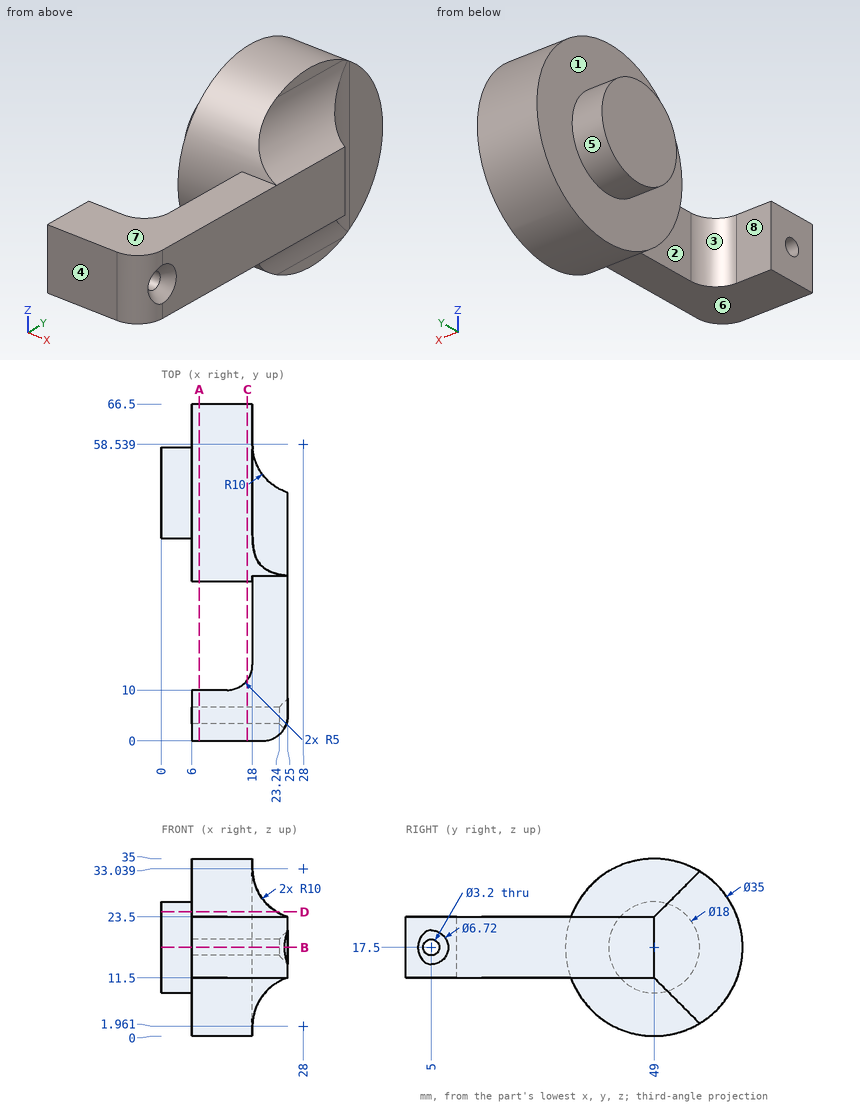
Source: three-view drawing plus pictorial views. Frame: mm from the lowest corner of the part. A direction names the side the tool comes from. Coordinates: 2 decimals unless noted, no trailing zeros. Order: outer loops, then holes, each group sorted by start corner. A loop starts at its lowest first (then second) coordinate and runs counter-clockwise, first axis right, second up. Notation, with made-up numbers: M -9,16 L 49,16 A27 ccw 49,41 Z; hole C 23,51 d9. An arc over 180 degrees is marked long. Answer in a Markdown table with one row per item.
(1) Section query D-D, the plane z = 24.5. Output: boundary loops of the cut face in (x, y).
Numbers:
| item | result |
|---|---|
| outline | M 0,43.34 L 6,43.34 L 6,32.96 L 22.8,32.96 L 22.8,50 A10 cw 18,58.54 L 18,65.04 L 6,65.04 L 6,54.66 L 0,54.66 Z |
(2) Draft query along Y for the marked faces 1, 2, 3 and 4. Return one class per face: pulls with the +Y half, pulls with the -Y half, needs draft (parallel to the pull), parting line crosses it, or undercut.
Numbers:
| item | result |
|---|---|
| face 1 | needs draft |
| face 2 | undercut |
| face 3 | undercut |
| face 4 | pulls with the -Y half |
(3) Section query C-C, the plane x = 17. Output: boundary loops of the cut face in (y, z), plus the area to 3 significant figures.
Numbers:
| item | result |
|---|---|
| outline | M 0,11.5 L 12,11.5 L 12,23.5 L 0,23.5 Z; C 49,17.5 d35; hole C 5,17.5 d3.2 |
| area | 1,100 mm^2 |
(4) Material intervals for line 1 (X direction, y = 59.5, z = 31); line 2 (Y direction, x = 3.25, z = 21.5); line 3 (X direction, y = 24.5, z = 17.5), sorted ascending. Write a range as [from, to].
Numbers:
| item | result |
|---|---|
| line 1 | x = [6, 18] |
| line 2 | y = [40.94, 57.06] |
| line 3 | x = [18, 25] |
(5) Section query B-B, the plane z = 17.5. Output: boundary loops of the cut face in (x, y).
Numbers:
| item | result |
|---|---|
| outline | M 0,40 L 6,40 L 6,31.5 L 18,31.5 L 18,15 A5 cw 13,10 L 6,10 L 6,6.6 L 23.24,6.6 L 25,8.36 L 25,49 A10 cw 18,58.54 L 18,66.5 L 6,66.5 L 6,58 L 0,58 Z; M 6,0 L 20,0 A5 ccw 24.26,2.38 L 23.24,3.4 L 6,3.4 Z |
(6) Access query for the marked faces 5, 6, 7 and 8. Directions: +Z, -Z, +X, -X, +Y, -Y. A direction counts if a zero-diameter tool reaches every point of the face in a straight line with its end or side. Return the directions, or none.
Numbers:
| item | result |
|---|---|
| face 5 | -X |
| face 6 | -Z, +X, -X, -Y |
| face 7 | +Z, +X, -X, -Y |
| face 8 | +Z, -Z, -X |
(7) Contact query for flat-ended pins moving along their axis: pin 1 Ø4 at (y, z) = (33.5, 10) entering from -X; pin 2 Ø5.5 at (x, y) = (16, 19.5) entering from +Z; pin 3 Ø6 at (x, z) = (18.5, 25) entering from +Y. Output: stop coordinate, or through.
Numbers:
| item | result |
|---|---|
| pin 1 | stops at x = 6 |
| pin 2 | stops at z = 23.5 |
| pin 3 | stops at y = 65.9 |
(8) Section query A-A, the plane x = 7.5. Output: boundary loops of the cut face in (y, z).
Numbers:
| item | result |
|---|---|
| outline | M 0,11.5 L 10,11.5 L 10,23.5 L 0,23.5 Z; C 49,17.5 d35; hole C 5,17.5 d3.2 |
